```python
from build123d import *

# Parameters (mm, degrees)
SKETCH_1_R          = 3.5
EXTRUDE_1_DEPTH     = 4
SKETCH_3_R          = 3.5
EXTRUDE_2_DEPTH     = 3.3
SKETCH_4_W          = 4.5
SKETCH_4_H          = 4.5
EXTRUDE_3_DEPTH     = 2.5
SKETCH_7_R          = 3.5
CUT_EXTRUDE_1_DEPTH = 10


with BuildPart() as part:
    # 草图1 → 凸台-拉伸1 (new body)
    with BuildSketch(Plane(origin=(0, 0, 0), x_dir=(1, 0, 0), z_dir=(0, 1, 0))):
        Circle(SKETCH_1_R)
        with BuildLine():
            Line((0.95, -1.2), (-0.95, -1.2))
            ThreePointArc((-0.95, -1.2), (-1.376776695, -1.376776695), (-1.2, -0.95))
            Line((-1.2, -0.95), (-1.2, 0.95))
            ThreePointArc((-1.2, 0.95), (-1.376776695, 1.376776695), (-0.95, 1.2))
            Line((-0.95, 1.2), (0.95, 1.2))
            ThreePointArc((0.95, 1.2), (1.376776695, 1.376776695), (1.2, 0.95))
            Line((1.2, 0.95), (1.2, -0.95))
            ThreePointArc((1.2, -0.95), (1.376776695, -1.376776695), (0.95, -1.2))
        make_face(mode=Mode.SUBTRACT)
    extrude(amount=EXTRUDE_1_DEPTH)

    # 草图3 → 凸台-拉伸2 (add)
    with BuildSketch(Plane(origin=(0, 4, 0), x_dir=(1, 0, 0), z_dir=(0, 1, 0))):
        Circle(SKETCH_3_R)
    extrude(amount=EXTRUDE_2_DEPTH)

    # 草图4 → 凸台-拉伸3 (add)
    with BuildSketch(Plane(origin=(0, 7.3, 0), x_dir=(1, 0, 0), z_dir=(0, 1, 0))):
        Rectangle(SKETCH_4_W, SKETCH_4_H)
    extrude(amount=EXTRUDE_3_DEPTH)

    # 草图5 → 旋转1 (revolve)
    with BuildSketch(Plane(origin=(0, 9.8, 0), x_dir=(1, 0, 0), z_dir=(0, 1, 0))):
        with BuildLine():
            Line((-2.75, 0), (-1.75, 0))
            ThreePointArc((-1.75, 0), (-2.25, -0.5), (-2.75, 0))
        make_face()
        with BuildLine():
            Line((1.75, 0), (2.75, 0))
            ThreePointArc((2.75, 0), (2.25, -0.5), (1.75, 0))
        make_face()
    revolve(axis=Axis((-2.75, 9.8, 0), (1, 0, 0)))

    # 草图6 → 旋转2 (revolve)
    with BuildSketch(Plane(origin=(0, 9.8, 0), x_dir=(1, 0, 0), z_dir=(0, 1, 0))):
        with BuildLine():
            Line((0, -2.75), (0, -1.75))
            ThreePointArc((0, -1.75), (-0.5, -2.25), (0, -2.75))
        make_face()
        with BuildLine():
            Line((0, 1.75), (0, 2.75))
            ThreePointArc((0, 2.75), (-0.5, 2.25), (0, 1.75))
        make_face()
    revolve(axis=Axis((0, 9.8, 2.75), (0, 0, -1)))

    # 草图7 → 切除-拉伸1 (cut)
    with BuildSketch(Plane(origin=(0, 9.8, 0), x_dir=(1, 0, 0), z_dir=(0, 1, 0))):
        Circle(SKETCH_7_R)
    extrude(amount=CUT_EXTRUDE_1_DEPTH, mode=Mode.SUBTRACT)


solid = part.part
```
Model file for the job. Use its own axes, mm. A direction names the side the tool comes from. Coordinates: 2 decimals unless noted, no trailing zeros. Order: outer loops, then holes, each group sorted by start corner. A loop starts at its lowest first (then second) coordinate and runs counter-clockwise, first axis right, second up. Notation, with made-up numbers: (-36.5, 67.5) -> (-14.5, 67.5) arc R21 cw to (-14.5, 78.5) -> close; hole circle Ø6 at (74, 64). An arc over 180 degrees is marked (long way). Answer as a JSON object with one key per item and string values. Group by question number.
1) Cut at D-D, the plane y = 5.5. Write the cut outline in (x, z), then the cut area to 3 significant figures.
2) Which spindle directions (+Z, -Z, +X, -X, +Y, -Y) get a long thin tool onto all of the face, cutting with end or side? Do faces 4 (the face through (0, 0, 2)), 5 (the face through (0, 2, 1.2)). Say none if no direction does.
3) Cut at B-B, the plane x = 0. Write the cut outline in (y, z), then the cut area to 3 significant figures.
4) Flat gauge pins, fed straight in: pin 1 (2 mm diameter, centred on x = -1, y = 8.5, fed in from +Z); pin 2 (0.8 mm diameter, centred on x = 0.5, y = 9, fed in from -Z); pin 3 (1.3 mm diameter, centred on y = 8.5, z = -0.5, fed in from -X). Where does each tip first touch, or does it go through?
5) Cut at C-C, the plane z = 0. Write the cut outline in (x, y), then the cut area to 3 significant figures.
6) Drill centre lines: L1, parallel to X at y = 9.25, z = 0.25; L2, parallel to Y at x = -0.5, z = 3.25; L3, parallel to Z at x = 0.5, y = 2.5. Where is each one in solid material? Low to high.
7) Pull direction Z, two halves, no side cores. Call faces 1 (the face through (0, 2, -1.2)), 2 (the face through (3.233, 3.599, 1.341)), 3 (the face through (0, 9.8, 0)): +Z half, -Z half, draft (parallel to the pull), parting line (faces both ways), or undercut.
8) Cut at A-A, the plane y = 1. Write the cut outline in (x, z), then the cut area to 3 significant figures.
Check values:
{
 "1": {"outline": "circle Ø7 at (0, 0)", "area": "38.5 mm²"},
 "2": {"face 4": "+Z, -Z, +X, -X, -Y", "face 5": "-Y"},
 "3": {"outline": "(0, -3.5) -> (7.3, -3.5) -> (7.3, -2.25) -> (9.3, -2.25) arc R0.5 ccw to (9.8, -2.75) -> (9.8, 2.75) arc R0.5 ccw to (9.3, 2.25) -> (7.3, 2.25) -> (7.3, 3.5) -> (0, 3.5) -> (0, 1.2) -> (4, 1.2) -> (4, -1.2) -> (0, -1.2) -> close", "area": "53.1 mm²"},
 "4": {"pin 1": "stops at z = 2.25", "pin 2": "stops at z = -2.25", "pin 3": "stops at x = -2.25"},
 "5": {"outline": "(-3.5, 0) -> (-1.2, 0) -> (-1.2, 4) -> (1.2, 4) -> (1.2, 0) -> (3.5, 0) -> (3.5, 7.3) -> (2.25, 7.3) -> (2.25, 9.3) arc R0.5 ccw to (2.75, 9.8) -> (-2.75, 9.8) arc R0.5 ccw to (-2.25, 9.3) -> (-2.25, 7.3) -> (-3.5, 7.3) -> close", "area": "53.1 mm²"},
 "6": {"L1": "x = -2.25 to 2.25", "L2": "y = 0 to 7.3", "L3": "z = -3.46 to -1.2, 1.2 to 3.46"},
 "7": {"face 1": "undercut", "face 2": "parting line", "face 3": "draft"},
 "8": {"outline": "circle Ø7 at (0, 0); hole (-1.2, -0.95) arc R0.25 ccw (long way) to (-0.95, -1.2) -> (0.95, -1.2) arc R0.25 ccw (long way) to (1.2, -0.95) -> (1.2, 0.95) arc R0.25 ccw (long way) to (0.95, 1.2) -> (-0.95, 1.2) arc R0.25 ccw (long way) to (-1.2, 0.95) -> close", "area": "32.1 mm²"}
}
